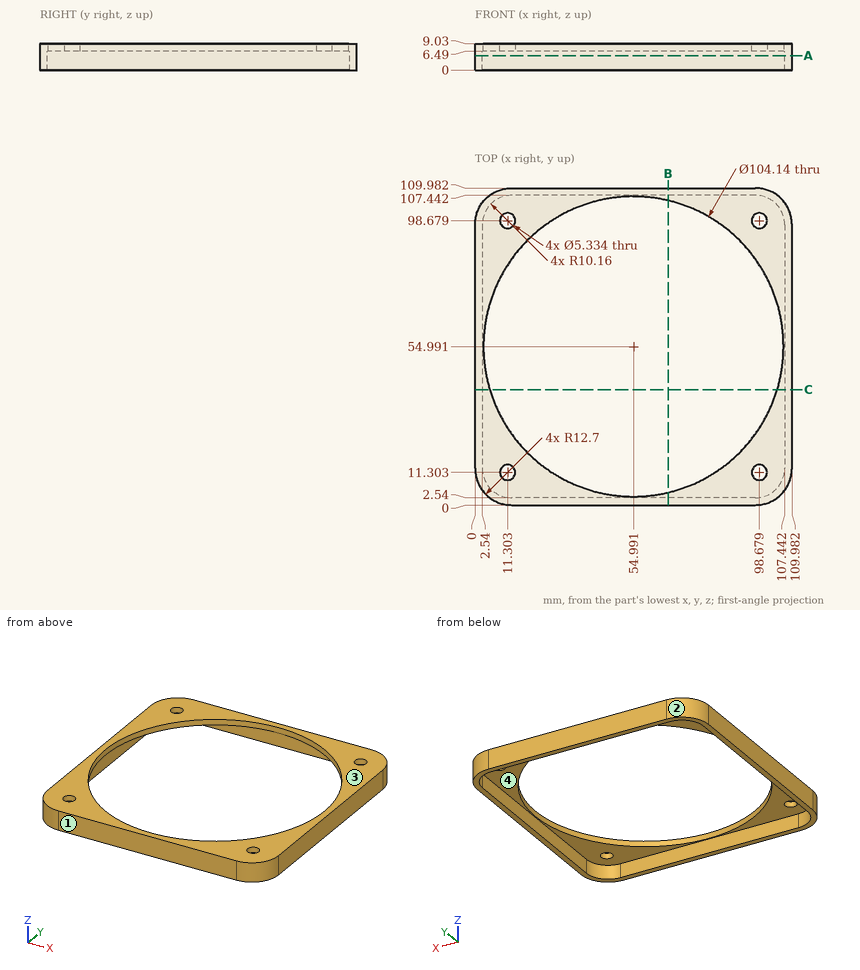
The figure shows three views and two pictorial views of one solid part (mm, origin at its lowest corner). Answer the questions. Give positions to 0.01 mm unless a question says otherwise; leave off trailing zeros. Write each loop counter-clockwise with the first axis right and the second up, starting at its lowest first coordinate (ties: lowest second). Pieces come first, ordered by that corner, then holes. Notation, with made-up numbers: M -6,26.5 L 10,26.5 A9 cw 10,39.5 Z; hole C -23.5,34.25 d3. An arc over 180 degrees is marked long. One line per item, written item: value. Start each with the question number.
(1) Find the intervals of material crossed by line 1 (Y direction, x = 45, z = 5.25); line 2 (X direction, y = 99.5, z = 6.75) (1 decimal), in increasing order.
(2) A flat-ended cylindrical pin translates along its axis: pin 1 Ø4.5 at (x, y) = (98.679, 11.303) entering from -Z. Find the tip coordinate at first contact, or state that the pin passes through.
(3) Find section A-A (z = 5). Determine the outline of the cut face in (x, y).
(4) Find section C-C (y = 40). Determine the outline of the cut face in (x, z), plus the area to 3 significant figures.
(5) Determine the mould class of the marked faces 1, 2, 3 and 4 for opening direction Y: pulls with the +Y half, pulls with the -Y half, needs draft (parallel to the pull), parting line crosses it, or undercut.
(6) Find section B-B (x = 67). Determine the outline of the cut face in (y, z) (1 decimal).
Results below:
1. line 1: y = 0 to 2.54, 107.44 to 109.98
1. line 2: x = 0.2 to 8.8, 13.8 to 28, 82 to 96.1, 101.2 to 109.8
2. pin 1: passes through
3. outline: M 0,12.7 A12.7 ccw 12.7,0 L 97.28,0 A12.7 ccw 109.98,12.7 L 109.98,97.28 A12.7 ccw 97.28,109.98 L 12.7,109.98 A12.7 ccw 0,97.28 Z; hole M 2.54,12.7 A10.16 ccw 12.7,2.54 L 97.28,2.54 A10.16 ccw 107.44,12.7 L 107.44,97.28 A10.16 ccw 97.28,107.44 L 12.7,107.44 A10.16 ccw 2.54,97.28 Z
4. outline: M 0,0 L 2.54,0 L 2.54,6.49 L 5.13,6.49 L 5.13,9.03 L 0,9.03 Z; M 104.86,6.49 L 107.44,6.49 L 107.44,0 L 109.98,0 L 109.98,9.03 L 104.86,9.03 Z
4. area: 59.0 mm^2
5. face 1: pulls with the -Y half
5. face 2: pulls with the +Y half
5. face 3: needs draft
5. face 4: undercut
6. outline: M 0,0 L 2.5,0 L 2.5,6.5 L 4.3,6.5 L 4.3,9 L 0,9 Z; M 105.7,6.5 L 107.4,6.5 L 107.4,0 L 110,0 L 110,9 L 105.7,9 Z
